from build123d import *

# Parameters (mm, degrees)
SKETCH1_R           = 1.5
BOSS_EXTRUDE1_DEPTH = 8.3
FILLET1_R           = 3


with BuildPart() as part:
    # Sketch1 → Boss-Extrude1 (new body)
    with BuildSketch(Plane(origin=(0, 0, 0), x_dir=(1, 0, 0), z_dir=(0, 1, 0))):
        with BuildLine():
            Line((0, 4), (30, 4))
            ThreePointArc((30, 4), (33.005515029, 2.639484686), (33.966505447, -0.516560296))
            Line((33.966505447, -0.516560296), (52.699163274, -11.331865335))
            Line((52.699163274, -11.331865335), (56.797239485, -10.233789123))
            Line((56.797239485, -10.233789123), (61.127366504, -12.733789123))
            Line((61.127366504, -12.733789123), (59.127366504, -16.197890739))
            ThreePointArc((59.127366504, -16.197890739), (56.69854107, -18.061594044), (53.663264889, -17.661992354))
            Line((53.663264889, -17.661992354), (30, -4))
            Line((30, -4), (0, -4))
            ThreePointArc((0, -4), (-4, 0), (0, 4))
        make_face()
        with Locations(Location((0, 0, 0), (0, 0, 90))):
            Circle(SKETCH1_R, mode=Mode.SUBTRACT)
        with Locations(Location((30, 0, 0), (0, 0, 90))):
            Circle(SKETCH1_R, mode=Mode.SUBTRACT)
    extrude(amount=BOSS_EXTRUDE1_DEPTH)

    # Fillet1
    fillet1_edges = [part.edges().sort_by_distance(p)[0] for p in [
        (52.699163274, 4.15, 11.331865335),
        (33.966505447, 4.15, 0.516560296),
    ]]
    fillet(fillet1_edges, radius=FILLET1_R)


solid = part.part
Work out the finished part from the listing and answer in its coordinate system (mm). A direction names the side the tool comes from. Coordinates: 2 decimals unless noted, no trailing zeros. Loops run counter-clockwise (first coordinate to the right, second up) from the corner with the lowest first, then second, coordinate; pieces in that order, holes last. Notation, with made-up numbers: (-37, 22.5) -> (-14, 22.5) arc R30 cw to (-14, 48.5) -> close; hole circle Ø7 at (43, 64.25). An arc over 180 degrees is marked (long way). Write each question's results on one line, items separated by ' | '. Start each with the question number.
1) Consider line 1 along Z through (x, y) = (30, 5.75); line 2 along X through (y, z) = (5.5, 0); line 3 along X through (y, z) = (0.5, -0.25). Determine where each line is inside the solid, lowest interval first.
2) Find section D-D on z = 2.5. Determine the outline of the cut face in (x, y), then the cut area to 3 significant figures.
3) For faces 1 (the flat face through (55.328, 4.092, 10.627)), 2 (the flat face through (60.14, 4.09, 14.44)), determine the directions among +Z, -Z, +X, -X, +Y, -Y from which every point of the face is accessible in a straight line to the end or side of a thin tool.
4) Find section C-C on x = 8. Determine the outline of the cut face in (y, z).
5) Find section A-A on z = 0. Determine the outline of the cut face in (x, y), then the cut area to 3 significant figures.
6) Find section B-B on y = 2.5. Determine the outline of the cut face in (x, z).
7) Flat-ended cylindrical pins translate along their axes: P1, Ø3, axis at x = 27, y = 1, coming from the +Z side; P2, Ø1.5, axis at x = 44, z = 4, coming from the -Y side; P3, Ø2, axis at y = 1, z = 14, coming from the +X side; P4, Ø4, axis at y = 1.5, z = 5.5, coming from the +X side. Find the tip coordinate at first contact, or state that the pin passes through.
8) The mould has two halves that part along X. Classify faces 3 (the cylindrical face through (28.513, 4.092, 0.195)), 4 (the flat face through (15, 4, 4)), 5 (the flat face through (42, 4.09, 10.93)), 6 (the cylindrical face through (34.42, 4.21, 0.45)): pulls with the +X half, pulls with the -X half, needs draft (parallel to the pull), parting line crosses it, or undercut.
Response values:
1) line 1: z = -4 to -1.5, 1.5 to 4 | line 2: x = -4 to -1.5, 1.5 to 28.5, 31.5 to 34.16 | line 3: x = -3.99 to -1.48, 1.48 to 28.52, 31.48 to 34.06
2) outline: (-3.12, 0) -> (37.4, 0) -> (37.4, 8.3) -> (-3.12, 8.3) -> close | area: 336 mm^2
3) face 1: -Z, +Y, -Y | face 2: +Z, +X, +Y, -Y
4) outline: (0, -4) -> (8.3, -4) -> (8.3, 4) -> (0, 4) -> close
5) outline: (-4, 0) -> (-1.5, 0) -> (-1.5, 8.3) -> (-4, 8.3) -> close; (1.5, 0) -> (28.5, 0) -> (28.5, 8.3) -> (1.5, 8.3) -> close; (31.5, 0) -> (34.16, 0) -> (34.16, 8.3) -> (31.5, 8.3) -> close | area: 267 mm^2
6) outline: (0, -4) -> (30, -4) arc R4 ccw to (33.93, -0.72) arc R3 cw to (35.39, 1.34) -> (51.62, 10.71) arc R3 cw to (53.9, 11.01) -> (56.8, 10.23) -> (61.13, 12.73) -> (59.13, 16.2) arc R4 ccw to (53.66, 17.66) -> (30, 4) -> (0, 4) arc R4 ccw to start; hole circle Ø3 at (0, 0); hole circle Ø3 at (30, 0)
7) P1: stops at z = 4 | P2: passes through | P3: stops at x = 60.97 | P4: stops at x = 46.06
8) face 3: undercut | face 4: needs draft | face 5: pulls with the -X half | face 6: pulls with the +X half
